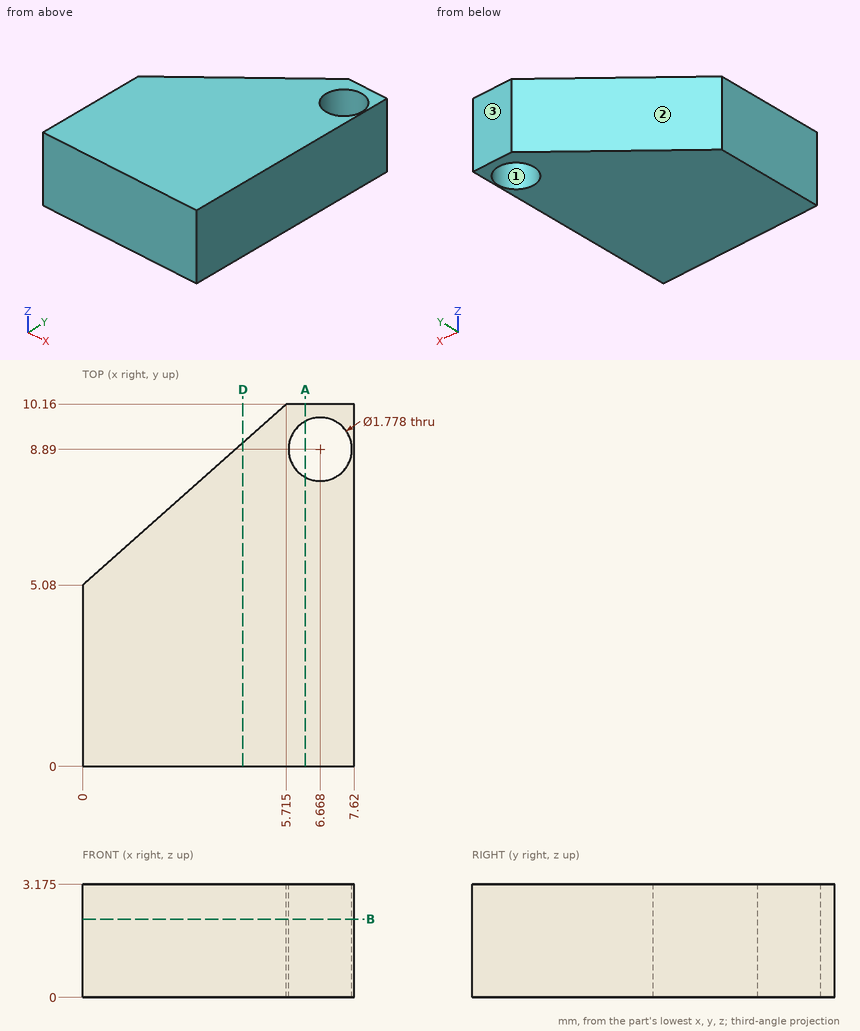
Geometry: see drawing. Coordinates: mm, zero at the bounding-box minimum. Give positions to 0.01 mm unless a question says otherwise; leave off trailing zeros. Loops run counter-clockwise (first coordinate to the right, second up) from the corner with the lowest first, then second, coordinate; pieces in that order, holes last. Notation, with made-up numbers: (-32, 3.25) - (19, 3.25) arc R22 ccw to (19, 15.25) - close; hole circle Ø10 at (88.25, 18). An arc over 180 degrees is marked (long way). One line per question, with ' | ' between items. Start each with the question number.
(1) Section query D-D on x = 4.5. Return loops of the section in (y, z) (1 decimal).
(2) Section query A-A on x = 6.25. Return loops of the section in (y, z) (1 decimal).
(3) Pull-direction query (X, two-part tool) for the marked faces 1, 2 and 3; classes: released by +X, released by -X, zero draft, split by the parting line, or undercut.
(4) Ray query, line 1 (Y direction, x = 6.5, z = 1.6); line 2 (Y direction, x = 5, z = 1.1) (1 decimal); line 3 (Y direction, x = 1, z = 2.8). Return the intervals inside material, ascending. Write a range as from..to.
(5) Contact query for flat-ended pins moving along their axis: pin 1 (2.5 mm diameter, centred on x = 6.67, y = 8.89, fed in from +Z) (1 decimal); pin 2 (1 mm diameter, centred on y = 6.5, z = 1, fed in from -X) (1 decimal); pin 3 (1.5 mm diameter, centred on x = 1.5, z = 2, fed in from +Y). Output: stop coordinate, or through.
(6) Section query B-B on z = 2.2. Return loops of the section in (x, y) (1 decimal).
The answers:
1) outline: (0, 0) - (9.1, 0) - (9.1, 3.2) - (0, 3.2) - close
2) outline: (0, 0) - (8.1, 0) - (8.1, 3.2) - (0, 3.2) - close; (9.7, 0) - (10.2, 0) - (10.2, 3.2) - (9.7, 3.2) - close
3) face 1: undercut | face 2: released by -X | face 3: zero draft
4) line 1: 0..8.02, 9.76..10.16 | line 2: 0..9.5 | line 3: 0..5.97
5) pin 1: z = 3.2 | pin 2: x = 1 | pin 3: y = 7.08
6) outline: (0, 0) - (7.6, 0) - (7.6, 10.2) - (5.7, 10.2) - (0, 5.1) - close; hole circle Ø1.8 at (6.7, 8.9)
